Geometry check sheet. Reference: the model listing, model coordinates, mm. Round coordinates to 2 decimals unless told otherwise and drop trailing zeros. Write each loop counter-clockwise with the first axis right and the second up, starting at its lowest first coordinate (ties: lowest second). Pieces come first, ordered by that corner, then holes. Notation, with made-up numbers: (7, 83.25) -> (27, 83.25) arc R11 cw to (27, 94.25) -> close; hole circle Ø9 at (79.25, 35.5). An arc over 180 degrees is marked (long way). Use a Markdown table: item, result.
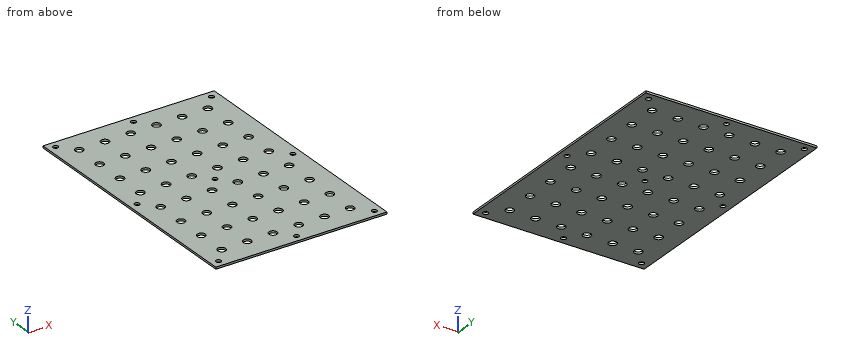
Autodesk Fusion 360 part; units mm, degrees
sketch "Sketch1" plane through (0, 0, 0) normal (0, 0, 1) x (1, 0, 0)
  line L0 (42.595, 63.475) -> (-42.595, 63.475)
  line L1 (-42.595, 63.475) -> (-42.595, -63.475)
  line L2 (-42.595, -63.475) -> (42.595, -63.475)
  line L3 (42.595, -63.475) -> (42.595, 63.475)
  line L4 (42.595, 63.475) -> (-42.595, -63.475) construction
  line L5 (-42.595, 63.475) -> (42.595, -63.475) construction
  line L6 (37.095, 57.275) -> (-37.095, 57.275)
  line L7 (-37.095, 57.275) -> (-37.095, -57.275)
  line L8 (-37.095, -57.275) -> (37.095, -57.275)
  line L9 (37.095, -57.275) -> (37.095, 57.275)
  line L10 (37.095, 57.275) -> (-37.095, -57.275) construction
  line L11 (-37.095, 57.275) -> (37.095, -57.275) construction
  line L12 (34.095, 54.275) -> (-34.095, 54.275)
  line L13 (-34.095, 54.275) -> (-34.095, -54.275)
  line L14 (-34.095, -54.275) -> (34.095, -54.275)
  line L15 (34.095, -54.275) -> (34.095, 54.275)
  line L16 (34.095, 54.275) -> (-34.095, -54.275) construction
  line L17 (-34.095, 54.275) -> (34.095, -54.275) construction
  dimension "d1" = 85.19
  dimension "d2" = 126.95
  dimension "d3" = 74.19
  dimension "d4" = 114.55
  dimension "d5" = 68.19
  dimension "d6" = 108.55
sketch "Sketch2" plane through (0, 0, 0) normal (0, 0, 1) x (1, 0, 0)
sketch "Sketch3" plane through (0, 0, 0) normal (0, 0, 1) x (1, 0, 0)
  line L0 (34.095, 54.275) -> (-34.095, 54.275)
  line L1 (-34.095, 54.275) -> (-34.095, -54.275)
  circle A0 centre (-32.095, 52.275) radius 2
  dimension "d7" = 2
extrude "Extrude1" add sketch "Sketch1" along normal blind 1 contours L0 L1 L2 L3 | L6 L7 L8 L9 | L12 L13 L14 L15
sketch "Sketch4" plane through (0, 0, 0) normal (0, 0, 1) x (1, 0, 0)
sketch "Sketch5" plane through (0, 0, 1) normal (0, 0, 1) x (-1, 0, 0)
  line L0 (-42.595, 63.475) -> (-42.595, -63.475)
  line L1 (-42.595, -63.475) -> (42.595, -63.475)
  line L2 (42.595, -63.475) -> (42.595, 63.475)
  line L3 (42.595, 63.475) -> (-42.595, 63.475)
  line L4 (-34.095, 54.275) -> (34.095, 54.275)
  line L5 (34.095, 54.275) -> (34.095, -54.275)
  line L6 (34.095, -54.275) -> (-34.095, -54.275)
  line L7 (-34.095, -54.275) -> (-34.095, 54.275)
  line L8 (-34.095, 54.275) -> (34.095, -54.275) construction
  line L9 (34.095, 54.275) -> (-34.095, -54.275) construction
  circle A0 centre (32.095, -52.275) radius 2
  dimension "d10" = 68.19
  dimension "d11" = 108.55
  dimension "d12" = 2
loft "Loft1" cut profiles "Sketch5", "Sketch3" section 1 contours A0 section 2 contours A0
pattern_linear "R-Pattern1" count 6 spacing 12.8 along (1, 0, 0) count 8 spacing 14.9286 along (0, -1, 0) of "Loft1"
sketch "Sketch6" plane through (0, 0, 1) normal (0, 0, 1) x (-1, 0, 0)
  circle A0 centre (0, 0) radius 1.5
  circle A1 centre (0, -59.81) radius 1.5
  circle A2 centre (0, 59.81) radius 1.5
  circle A3 centre (38.77, -59.81) radius 1.5
  circle A4 centre (38.77, 0) radius 1.5
  circle A5 centre (38.77, 59.81) radius 1.5
  circle A6 centre (-38.77, 0) radius 1.5
  circle A7 centre (-38.77, 59.81) radius 1.5
  circle A8 centre (-38.77, -59.81) radius 1.5
  dimension "d17" = 3
  dimension "d18" = 59.81
  dimension "d19" = 3
  dimension "d20" = 59.81
  dimension "d21" = 3
  dimension "d23" = 3
  dimension "d24" = 3
  dimension "d25" = 59.81
  dimension "d26" = 3
  dimension "d28" = 3
  dimension "d29" = 3
  dimension "d30" = 59.81
  dimension "d31" = 3
hole "Hole1" at (-38.77, 59.81, 1) at (0, 59.81, 1) at (38.77, 59.81, 1) at (38.77, 0, 1) at (-38.77, 0, 1) at (-38.77, -59.81, 1) at (0, -59.81, 1) at (38.77, -59.81, 1) at (0, 0, 1) direction (0, 0, -1) diameter 2.529 depth 14 tip angle 180
(1) Section check B-B on x = 0. Record the cut outline in (y, z) (1 decimal), plus the area to 3 significant figures.
A:
| item | result |
|---|---|
| outline | (-63.5, 0) -> (-61.1, 0) -> (-61.1, 1) -> (-63.5, 1) -> close; (-58.5, 0) -> (-1.3, 0) -> (-1.3, 1) -> (-58.5, 1) -> close; (1.3, 0) -> (58.5, 0) -> (58.5, 1) -> (1.3, 1) -> close; (61.1, 0) -> (63.5, 0) -> (63.5, 1) -> (61.1, 1) -> close |
| area | 119 mm2 |
(2) Section check A-A on y = 0. Record the cut outline in (x, z) (1 decimal).
A:
| item | result |
|---|---|
| outline | (-42.6, 0) -> (-40, 0) -> (-40, 1) -> (-42.6, 1) -> close; (-37.5, 0) -> (-1.3, 0) -> (-1.3, 1) -> (-37.5, 1) -> close; (1.3, 0) -> (37.5, 0) -> (37.5, 1) -> (1.3, 1) -> close; (40, 0) -> (42.6, 0) -> (42.6, 1) -> (40, 1) -> close |
(3) Thickness scan on line 1 (Y direction, x = -39, z = 0.35) (3 decimals); line 2 (Y direction, x = 0, z = 0.65) (1 decimal). Record the ranges inside material, lowest first.
A:
| item | result |
|---|---|
| line 1 | y = -63.475 to -61.053, -58.567 to -1.243, 1.243 to 58.567, 61.053 to 63.475 |
| line 2 | y = -63.5 to -61.1, -58.5 to -1.3, 1.3 to 58.5, 61.1 to 63.5 |
(4) Section check C-C on z = 0.5. State how many separate pieces and enclosed holes the cut face has, plus the area to 3 significant figures.
A:
| item | result |
|---|---|
| separate pieces | 1 |
| enclosed holes | 57 |
| area | 10,200 mm2 |
